from build123d import *

# Parameters (mm, degrees)
BOSS_EXTRUDE1_DEPTH = 10
FILLET1_R           = 2


with BuildPart() as part:
    # Sketch1 → Boss-Extrude1 (new body)
    with BuildSketch(Plane(origin=(0, 0, 0), x_dir=(1, 0, 0), z_dir=(0, 1, 0))):
        Polygon((100, -50), (100, 50), (85, 50), (85, 32), (37, 32), (37, 50), (0, 50), (0, -50), (37, -50), (37, -32), (85, -32), (85, -50), align=None)
    extrude(amount=BOSS_EXTRUDE1_DEPTH)

    # Fillet1
    fillet1_edges = [part.edges().sort_by_distance(p)[0] for p in [
        (61, 0, 32),
        (37, 0, 41),
        (100, 10, 0),
        (18.5, 0, 50),
        (0, 0, 0),
        (18.5, 0, -50),
        (37, 0, -41),
        (61, 0, -32),
        (85, 0, -41),
        (92.5, 0, -50),
        (100, 0, 0),
        (92.5, 0, 50),
        (85, 0, 41),
        (92.5, 10, -50),
        (85, 5, 32),
        (37, 5, 32),
        (85, 10, -41),
        (0, 5, 50),
        (0, 5, -50),
        (37, 5, -50),
        (37, 5, -32),
        (85, 5, -32),
        (85, 5, -50),
        (100, 5, -50),
        (100, 5, 50),
        (85, 5, 50),
        (61, 10, -32),
        (37, 10, -41),
        (18.5, 10, -50),
        (0, 10, 0),
        (18.5, 10, 50),
        (37, 10, 41),
        (61, 10, 32),
        (85, 10, 41),
        (92.5, 10, 50),
    ]]
    fillet(fillet1_edges, radius=FILLET1_R)


solid = part.part
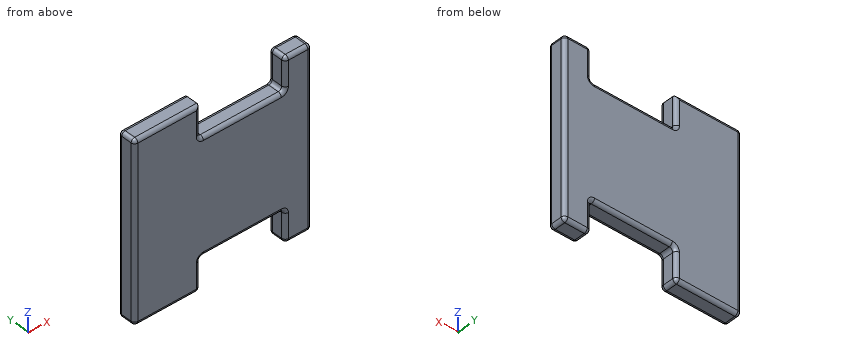
Input: part model. Units: mm. Frame: model coordinates. Round coordinates to 2 decimals unless told otherwise and drop trailing zeros. Order: outer loops, then holes, each group sorted by start corner. A loop starts at its lowest first (then second) coordinate and runs counter-clockwise, first axis right, second up. Notation, with made-up numbers: (26.25, 31) - (31.25, 31) arc R24 ccw to (31.25, 51) - close; hole circle Ø7 at (-10, 9.25). An arc over 180 degrees is marked (long way). Answer as a JSON object with one key per item and string values. Group by question number.
(1) Cut plane A-A (z = -41). Return loops of the section in (x, y), then the cut area to 3 significant figures.
(2) Pin query (flat end, axial travel): P1, Ø3, axis at x = 72, y = 6, coming from the +Z side; P2, Ø5, axis at x = 58, y = 5, coming from the -Z side. Return the tip coordinate at first contact, or that it passes through.
(3) Material intervals for probe 1 along X at (y, z) = (6.75, -43.5); probe 2 along Z at (x, y) = (57, 4.75); probe 3 along Y at (x, z) = (86.5, 44), sorted ascending. Write a range as from..to.
(4) Cut plane C-C (y = 5.25). Return loops of the section in (x, z), then the cut area to 3 significant figures.
(5) Cut plane B-B (x = 62). Return loops of the section in (y, z), then the cut area to 3 significant figures.
Here are the results:
{
 "1": {"outline": "(0, 2) arc R2 ccw to (2, 0) - (35, 0) arc R2 ccw to (37, 2) - (37, 8) arc R2 ccw to (35, 10) - (2, 10) arc R2 ccw to (0, 8) - close; (85, 2) arc R2 ccw to (87, 0) - (98, 0) arc R2 ccw to (100, 2) - (100, 8) arc R2 ccw to (98, 10) - (87, 10) arc R2 ccw to (85, 8) - close", "area": "513 mm^2"},
 "2": {"P1": "stops at z = 32", "P2": "stops at z = -32"},
 "3": {"probe 1": "x = 0..37, 85..100", "probe 2": "z = -32..32", "probe 3": "y = 0.06..9.94"},
 "4": {"outline": "(0, -48) arc R2 ccw to (2, -50) - (35, -50) arc R2 ccw to (37, -48) - (37, -34) arc R2 cw to (39, -32) - (83, -32) arc R2 cw to (85, -34) - (85, -48) arc R2 ccw to (87, -50) - (98, -50) arc R2 ccw to (100, -48) - (100, 48) arc R2 ccw to (98, 50) - (87, 50) arc R2 ccw to (85, 48) - (85, 34) arc R2 cw to (83, 32) - (39, 32) arc R2 cw to (37, 34) - (37, 50) - (2, 50) arc R2 ccw to (0, 48) - close", "area": "8,270 mm^2"},
 "5": {"outline": "(0, -30) arc R2 ccw to (2, -32) - (8, -32) arc R2 ccw to (10, -30) - (10, 30) arc R2 ccw to (8, 32) - (2, 32) arc R2 ccw to (0, 30) - close", "area": "637 mm^2"}
}
